Autodesk Inventor part; units mm, degrees
ref_plane "YZ Plane" through (0, 0, 0) normal (1, 0, 0) x (0, 1, 0)
ref_plane "XZ Plane" through (0, 0, 0) normal (0, 1, 0) x (-1, 0, 0)
ref_plane "XY Plane" through (0, 0, 0) normal (0, 0, 1) x (1, 0, 0)
sketch "Sketch1" plane through (0, 0, 0) normal (0, 0, 1) x (1, 0, 0)
  line L0 (6.35, 3.6662) -> (6.35, -3.6662)
  line L1 (6.35, -3.6662) -> (0, -7.3323)
  line L2 (0, -7.3323) -> (-6.35, -3.6662)
  line L3 (-6.35, -3.6662) -> (-6.35, 3.6662)
  line L4 (-6.35, 3.6662) -> (0, 7.3323)
  line L5 (0, 7.3323) -> (6.35, 3.6662)
  circle A0 centre (0, 0) radius 1.4224
  dimension "d0" = 12.7
  dimension "d3" = 2.8448
extrude "Extrusion1" add sketch "Sketch1" along normal mid plane 38.1
properties part number "PIVOT,SHAFT,HEX,0.500in" material "Aluminum 6061"
The listing builds one solid part. Answer for the finished solid, in the listing's coordinates (mm). Give positions to 0.01 mm unless a question says otherwise; leave off trailing zeros. Loops run counter-clockwise (first coordinate to the right, second up) from the corner with the lowest first, then second, coordinate; pieces in that order, holes last. Notation, with made-up numbers: (59, 29.25) - (116, 29.25) arc R24 ccw to (116, 39.25) - close; hole circle Ø5 at (-27.5, 50). An arc over 180 degrees is marked (long way). Write each question's results on one line, items separated by ' | '.
1. Find section A-A, the plane z = 0. Write down the section's boundary in (x, y), then the cut area to 3 significant figures.
Resolved:
outline: (-6.35, -3.67) - (0, -7.33) - (6.35, -3.67) - (6.35, 3.67) - (0, 7.33) - (-6.35, 3.67) - close; hole circle Ø2.84 at (0, 0) | area: 133 mm^2
2. Consider probe 1 along Y at (x, z) = (0, 11); probe 2 along Y at (x, z) = (1, -9); probe 3 along X at (y, z) = (-1.25, -9). Determine where each line is inside the solid, lowest interval first. Write a range as from..to.
Resolved:
probe 1: y = -7.33..-1.42, 1.42..7.33 | probe 2: y = -6.75..-1.01, 1.01..6.75 | probe 3: x = -6.35..-0.68, 0.68..6.35
3. Find section B-B, the plane x = 0.75. Write down the section's boundary in (y, z), then the cut area to 3 significant figures.
Resolved:
outline: (-6.9, -19.05) - (-1.21, -19.05) - (-1.21, 19.05) - (-6.9, 19.05) - close; (1.21, -19.05) - (6.9, -19.05) - (6.9, 19.05) - (1.21, 19.05) - close | area: 434 mm^2
4. Find section C-C, the plane y = 4.75. Write down the section's boundary in (x, z).
Resolved:
outline: (-4.47, -19.05) - (4.47, -19.05) - (4.47, 19.05) - (-4.47, 19.05) - close
5. For a pull along Y with two mould halves and no side action, classify faces 1 (the face through (3.131, 5.525, -0.267)), 2 (the face through (0, -2, -19.05)), 3 (the face through (-3.131, -5.525, -0.267)), 4 (the face through (-0.31, 1.39, -0.27)) as +Y half, -Y half, draft (parallel to the pull), parting line (faces both ways), or undercut.
Resolved:
face 1: +Y half | face 2: draft | face 3: -Y half | face 4: undercut
6. Find section D-D, the plane x = 2.75. Write down the section's boundary in (y, z).
Resolved:
outline: (-5.74, -19.05) - (5.74, -19.05) - (5.74, 19.05) - (-5.74, 19.05) - close
7. Flat-ended cylindrical pins translate along their axes: P1, Ø4, axis at x = 2.5, z = -9.5, coming from the -Y side; P2, Ø6, axis at x = -1.5, z = 13, coming from the +Y side; P3, Ø6, axis at x = 2, z = -4, coming from the -Y side. Find the tip coordinate at first contact, or state that the pin passes through.
Resolved:
P1: stops at y = -7.04 | P2: stops at y = 7.33 | P3: stops at y = -7.33
